For this review, take the finished solid that the model builds, in its own axes (mm). Round coordinates to 2 decimals unless told otherwise and drop trailing zeros. Write each loop counter-clockwise with the first axis right and the second up, starting at its lowest first coordinate (ties: lowest second). Pieces come first, ordered by that corner, then holes.
from build123d import *

# Parameters (mm, degrees)
BOSS_EXTRUDE4_DEPTH = 1.9
SKETCH7_W           = 5.428932188
SKETCH7_H           = 2
BOSS_EXTRUDE5_DEPTH = 0.95


with BuildPart() as part:
    # Sketch6 → Boss-Extrude4 (new body)
    with BuildSketch(Plane(origin=(0, 0, 0), x_dir=(1, 0, 0), z_dir=(0, 1, 0))):
        with BuildLine():
            ThreePointArc((-12.5, -192.5), (0, -202.747548784), (12.5, -192.5))
            Line((12.5, -192.5), (12.5, 22.5))
            Line((12.5, 22.5), (7.071067812, 22.5))
            ThreePointArc((7.071067812, 22.5), (7.5, 20), (7.071067812, 17.5))
            ThreePointArc((7.071067812, 17.5), (7.5, 15), (7.071067812, 12.5))
            ThreePointArc((7.071067812, 12.5), (7.5, 10), (7.071067812, 7.5))
            ThreePointArc((7.071067812, 7.5), (7.5, 5), (7.071067812, 2.5))
            ThreePointArc((7.071067812, 2.5), (7.5, 0), (7.071067812, -2.5))
            ThreePointArc((7.071067812, -2.5), (7.5, -5), (7.071067812, -7.5))
            ThreePointArc((7.071067812, -7.5), (7.5, -10), (7.071067812, -12.5))
            ThreePointArc((7.071067812, -12.5), (7.5, -15), (7.071067812, -17.5))
            ThreePointArc((7.071067812, -17.5), (7.5, -20), (7.071067812, -22.5))
            ThreePointArc((7.071067812, -22.5), (7.5, -25), (7.071067812, -27.5))
            ThreePointArc((7.071067812, -27.5), (7.5, -30), (7.071067812, -32.5))
            ThreePointArc((7.071067812, -32.5), (0, -42.5), (-7.071067812, -32.5))
            ThreePointArc((-7.071067812, -32.5), (-7.5, -30), (-7.071067812, -27.5))
            ThreePointArc((-7.071067812, -27.5), (-7.5, -25), (-7.071067812, -22.5))
            ThreePointArc((-7.071067812, -22.5), (-7.5, -20), (-7.071067812, -17.5))
            ThreePointArc((-7.071067812, -17.5), (-7.5, -15), (-7.071067812, -12.5))
            ThreePointArc((-7.071067812, -12.5), (-7.5, -10), (-7.071067812, -7.5))
            ThreePointArc((-7.071067812, -7.5), (-7.5, -5), (-7.071067812, -2.5))
            ThreePointArc((-7.071067812, -2.5), (-7.5, 0), (-7.071067812, 2.5))
            ThreePointArc((-7.071067812, 2.5), (-7.5, 5), (-7.071067812, 7.5))
            ThreePointArc((-7.071067812, 7.5), (-7.5, 10), (-7.071067812, 12.5))
            ThreePointArc((-7.071067812, 12.5), (-7.5, 15), (-7.071067812, 17.5))
            ThreePointArc((-7.071067812, 17.5), (-7.5, 20), (-7.071067812, 22.5))
            Line((-7.071067812, 22.5), (-12.5, 22.5))
            Line((-12.5, 22.5), (-12.5, -192.5))
        make_face()
        with BuildLine():
            ThreePointArc((7.071067812, -57.5), (7.5, -60), (7.071067812, -62.5))
            ThreePointArc((7.071067812, -62.5), (7.5, -65), (7.071067812, -67.5))
            ThreePointArc((7.071067812, -67.5), (7.5, -70), (7.071067812, -72.5))
            ThreePointArc((7.071067812, -72.5), (7.5, -75), (7.071067812, -77.5))
            ThreePointArc((7.071067812, -77.5), (7.5, -80), (7.071067812, -82.5))
            ThreePointArc((7.071067812, -82.5), (7.5, -85), (7.071067812, -87.5))
            ThreePointArc((7.071067812, -87.5), (7.5, -90), (7.071067812, -92.5))
            ThreePointArc((7.071067812, -92.5), (7.5, -95), (7.071067812, -97.5))
            ThreePointArc((7.071067812, -97.5), (7.5, -100), (7.071067812, -102.5))
            ThreePointArc((7.071067812, -102.5), (7.5, -105), (7.071067812, -107.5))
            ThreePointArc((7.071067812, -107.5), (7.5, -110), (7.071067812, -112.5))
            ThreePointArc((7.071067812, -112.5), (7.5, -115), (7.071067812, -117.5))
            ThreePointArc((7.071067812, -117.5), (7.5, -120), (7.071067812, -122.5))
            ThreePointArc((7.071067812, -122.5), (7.5, -125), (7.071067812, -127.5))
            ThreePointArc((7.071067812, -127.5), (0, -137.5), (-7.071067812, -127.5))
            ThreePointArc((-7.071067812, -127.5), (-7.5, -125), (-7.071067812, -122.5))
            ThreePointArc((-7.071067812, -122.5), (-7.5, -120), (-7.071067812, -117.5))
            ThreePointArc((-7.071067812, -117.5), (-7.5, -115), (-7.071067812, -112.5))
            ThreePointArc((-7.071067812, -112.5), (-7.5, -110), (-7.071067812, -107.5))
            ThreePointArc((-7.071067812, -107.5), (-7.5, -105), (-7.071067812, -102.5))
            ThreePointArc((-7.071067812, -102.5), (-7.5, -100), (-7.071067812, -97.5))
            ThreePointArc((-7.071067812, -97.5), (-7.5, -95), (-7.071067812, -92.5))
            ThreePointArc((-7.071067812, -92.5), (-7.5, -90), (-7.071067812, -87.5))
            ThreePointArc((-7.071067812, -87.5), (-7.5, -85), (-7.071067812, -82.5))
            ThreePointArc((-7.071067812, -82.5), (-7.5, -80), (-7.071067812, -77.5))
            ThreePointArc((-7.071067812, -77.5), (-7.5, -75), (-7.071067812, -72.5))
            ThreePointArc((-7.071067812, -72.5), (-7.5, -70), (-7.071067812, -67.5))
            ThreePointArc((-7.071067812, -67.5), (-7.5, -65), (-7.071067812, -62.5))
            ThreePointArc((-7.071067812, -62.5), (-7.5, -60), (-7.071067812, -57.5))
            ThreePointArc((-7.071067812, -57.5), (0, -47.5), (7.071067812, -57.5))
        make_face(mode=Mode.SUBTRACT)
        with BuildLine():
            ThreePointArc((7.071067812, -152.5), (7.5, -155), (7.071067812, -157.5))
            ThreePointArc((7.071067812, -157.5), (7.5, -160), (7.071067812, -162.5))
            ThreePointArc((7.071067812, -162.5), (7.5, -165), (7.071067812, -167.5))
            ThreePointArc((7.071067812, -167.5), (7.5, -170), (7.071067812, -172.5))
            ThreePointArc((7.071067812, -172.5), (7.5, -175), (7.071067812, -177.5))
            ThreePointArc((7.071067812, -177.5), (7.5, -180), (7.071067812, -182.5))
            ThreePointArc((7.071067812, -182.5), (7.5, -185), (7.071067812, -187.5))
            ThreePointArc((7.071067812, -187.5), (0, -197.5), (-7.071067812, -187.5))
            ThreePointArc((-7.071067812, -187.5), (-7.5, -185), (-7.071067812, -182.5))
            ThreePointArc((-7.071067812, -182.5), (-7.5, -180), (-7.071067812, -177.5))
            ThreePointArc((-7.071067812, -177.5), (-7.5, -175), (-7.071067812, -172.5))
            ThreePointArc((-7.071067812, -172.5), (-7.5, -170), (-7.071067812, -167.5))
            ThreePointArc((-7.071067812, -167.5), (-7.5, -165), (-7.071067812, -162.5))
            ThreePointArc((-7.071067812, -162.5), (-7.5, -160), (-7.071067812, -157.5))
            ThreePointArc((-7.071067812, -157.5), (-7.5, -155), (-7.071067812, -152.5))
            ThreePointArc((-7.071067812, -152.5), (0, -142.5), (7.071067812, -152.5))
        make_face(mode=Mode.SUBTRACT)
    extrude(amount=BOSS_EXTRUDE4_DEPTH)

    # Sketch7 → Boss-Extrude5 (add)
    with BuildSketch(Plane(origin=(0, 0, 0), x_dir=(1, 0, 0), z_dir=(0, 1, 0))):
        with Locations((-9.785533906, 23.5)):
            Rectangle(SKETCH7_W, SKETCH7_H)
        with Locations((9.785533906, 23.5)):
            Rectangle(SKETCH7_W, SKETCH7_H)
    extrude(amount=BOSS_EXTRUDE5_DEPTH)


solid = part.part
(1) We need section A-A, the plane z = 55. Give the boundary of the cut face in (x, y).
Geometry check:
outline: (-12.5, 0) - (-7.5, 0) - (-7.5, 1.9) - (-12.5, 1.9) - close; (7.5, 0) - (12.5, 0) - (12.5, 1.9) - (7.5, 1.9) - close
(2) For pin 1 Ø1 at (x, y) = (9, 1) entering from -Z; pin 2 Ø1 at (x, z) = (-9.5, -23.5) entering from +Y; pin 3 Ø1 at (x, y) = (-10.5, 1.5) entering from -Z, all flat-tipped, find the tip position at first contact; note any pin that passes through.
Geometry check:
pin 1: stops at z = -24.5
pin 2: stops at y = 0.95
pin 3: stops at z = -22.5
(3) Mouldability with a two-part tool opening along Z and no side actions: class faces 1 (the face through (0.201, 0.937, 137.497)), 2 (the face through (-0.245, 0.937, 202.745)), 3 (the face through (-0.201, 0.937, 47.503)), 4 (the face through (-9, 0, 88)) as pulls with the +Z half, pulls with the -Z half, needs draft (parallel to the pull), parting line crosses it, or undercut.
Geometry check:
face 1: undercut
face 2: pulls with the +Z half
face 3: undercut
face 4: needs draft
(4) We need section D-D, the plane z = 14.5. Give the boundary of the cut face in (x, y).
Geometry check:
outline: (-12.5, 0) - (-7.48, 0) - (-7.48, 1.9) - (-12.5, 1.9) - close; (7.48, 0) - (12.5, 0) - (12.5, 1.9) - (7.48, 1.9) - close
(5) For line 1 along X through (y, z) = (0.75, 185); line 2 along Z through (x, y) = (-3.75, 0.8); line 3 along Z through (x, y) = (3.5, 1.1), list the stretches that pass through material, from the lowest coordinate up.
Geometry check:
line 1: x = -12.5 to -7.5, 7.5 to 12.5
line 2: z = 41.5 to 48.5, 136.5 to 143.5, 196.5 to 202.18
line 3: z = 41.63 to 48.37, 136.63 to 143.37, 196.63 to 202.26
(6) We need section B-B, the plane x = 0. Give the boundary of the cut face in (y, z), and give its area (3 significant figures).
Geometry check:
outline: (0, 42.5) - (1.9, 42.5) - (1.9, 47.5) - (0, 47.5) - close; (0, 137.5) - (1.9, 137.5) - (1.9, 142.5) - (0, 142.5) - close; (0, 197.5) - (1.9, 197.5) - (1.9, 202.75) - (0, 202.75) - close
area: 29.0 mm2
(7) We need section C-C, the plane y = 1.6. State how many separate pieces and enclosed holes the cut face has, and give its area (3 significant figures).
Geometry check:
separate pieces: 1
enclosed holes: 2
area: 2,590 mm2
